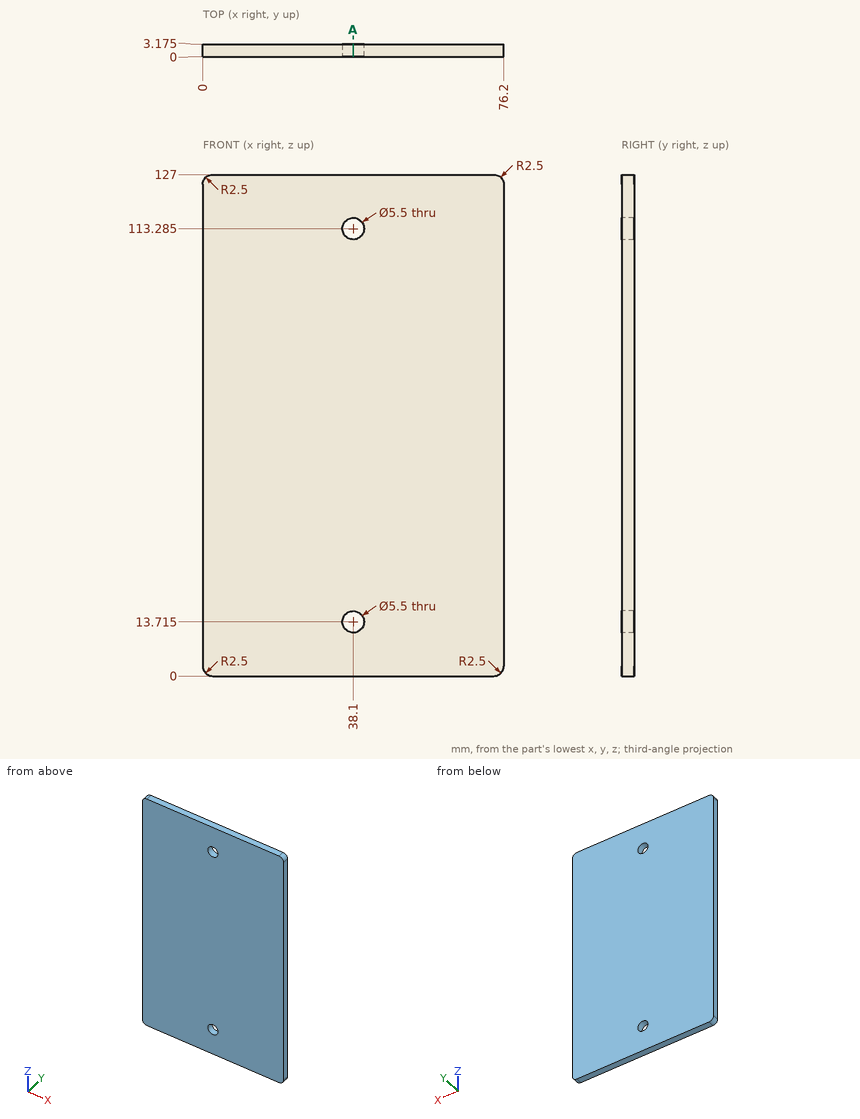
Print and shaded views of the part. All mm, measured from the part's lowest x, y and z. Coordinates: 2 decimals unless noted, no trailing zeros. Write each loop counter-clockwise with the first axis right and the second up, starting at its lowest first coordinate (ties: lowest second). Pieces come first, ordered by that corner, then holes. Notation, with made-up numbers: (-22.75, 2.25) -> (23.25, 2.25) arc R31 ccw to (23.25, 32.25) -> close; hole circle Ø10 at (68.25, -35.5). An arc over 180 degrees is marked (long way). Use CSV: the item, a comma, the result in double quotes. Start each with the question number.
Q1. Cut at A-A, the plane x = 38.1. List the corners of the cut face in (y, z) (3 decimals).
Q2. Drill centre lines: probe 1 along Z at (x, y) = (38.1, 2.3) (3 decimals); probe 2 along Z at (x, y) = (37, 1); probe 3 along X at (y, z) = (2.25, 12). Where is each one in solid material? Low to high.
Q3. Flat gauge pin, fed straight in: pin 1 Ø5 at (x, z) = (38.1, 13.715) entering from +Y. Where does the tip first touch, or does it go through?
Checked values:
1,outline,"(0, 0) -> (3.175, 0) -> (3.175, 10.965) -> (0, 10.965) -> close; (0, 16.465) -> (3.175, 16.465) -> (3.175, 110.535) -> (0, 110.535) -> close; (0, 116.035) -> (3.175, 116.035) -> (3.175, 127) -> (0, 127) -> close"
2,probe 1,"z = 0 to 10.965, 16.465 to 110.535, 116.035 to 127"
2,probe 2,"z = 0 to 11.19, 16.24 to 110.76, 115.81 to 127"
2,probe 3,"x = 0 to 35.95, 40.25 to 76.2"
3,pin 1,"passes through"
